Source: CAD feature listing. Evaluate the final solid. Frame: model axes, mm. A direction names the side the tool comes from. Give positions to 0.01 mm unless a question says otherwise; leave off trailing zeros. Order: outer loops, then holes, each group sorted by start corner. A loop starts at its lowest first (then second) coordinate and runs counter-clockwise, first axis right, second up. Notation, with made-up numbers: (1, 84) -> (6, 84) arc R18 ccw to (6, 117) -> close; hole circle Ø8 at (76, 42). An arc over 180 degrees is marked (long way). Use CSV: the item, a comma, the result in double quotes.
```python
from build123d import *

# Parameters (mm, degrees)
SKETCH1_W           = 80
SKETCH1_H           = 80
BOSS_EXTRUDE2_DEPTH = 10
CUT_EXTRUDE2_DEPTH  = 14
CUT_EXTRUDE3_DEPTH  = 14
CUT_EXTRUDE4_DEPTH  = 5
SCALE2_SCALE        = 0.1


with BuildPart() as part:
    # Sketch1 → Boss-Extrude2 (new body)
    with BuildSketch(Plane(origin=(0, 0, 0), x_dir=(1, 0, 0), z_dir=(0, 1, 0))):
        Rectangle(SKETCH1_W, SKETCH1_H)
    extrude(amount=BOSS_EXTRUDE2_DEPTH)

    # Sketch1<8> → Cut-Extrude2 (cut)
    with BuildSketch(Plane(origin=(0, 0, 0), x_dir=(1, 0, 0), z_dir=(0, 1, 0))):
        with BuildLine():
            Line((25, 40), (-25, 40))
            Line((-25, 40), (-25, 31.971455811))
            ThreePointArc((-25, 31.971455811), (-35.374629105, 30), (-25, 28.028544189))
            Line((-25, 28.028544189), (-25, 12.5))
            Line((-25, 12.5), (25, 12.5))
            Line((25, 12.5), (25, 28.028544189))
            ThreePointArc((25, 28.028544189), (35.374629105, 30), (25, 31.971455811))
            Line((25, 31.971455811), (25, 40))
        make_face()
    extrude(amount=CUT_EXTRUDE2_DEPTH, mode=Mode.SUBTRACT)

    # Sketch4 → Cut-Extrude3 (cut)
    with BuildSketch(Plane.XZ):
        Polygon((40, 40), (-40, 40), (-40, 25), (-38, 25), (38, 25), (40, 25), align=None)
    extrude(amount=-CUT_EXTRUDE3_DEPTH, mode=Mode.SUBTRACT)

    # Sketch4<4> → Cut-Extrude4 (cut)
    with BuildSketch(Plane.XZ):
        with BuildLine():
            Line((38, 25), (-38, 25))
            Line((-38, 25), (-38, -38))
            Line((-38, -38), (-27, -38))
            Line((-27, -38), (-25, -38))
            Line((-25, -38), (-25, -31.971455811))
            ThreePointArc((-25, -31.971455811), (-35.374629105, -30), (-25, -28.028544189))
            Line((-25, -28.028544189), (-25, -12.5))
            Line((-25, -12.5), (25, -12.5))
            Line((25, -12.5), (25, -28.028544189))
            ThreePointArc((25, -28.028544189), (35.374629105, -30), (25, -31.971455811))
            Line((25, -31.971455811), (25, -38))
            Line((25, -38), (27, -38))
            Line((27, -38), (38, -38))
            Line((38, -38), (38, 25))
        make_face()
    extrude(amount=-CUT_EXTRUDE4_DEPTH, mode=Mode.SUBTRACT)


with BuildPart() as part_1:
    # Scale2: scaled about (0, 7.105810112, -0.378714582)
    add(part.part.scale(SCALE2_SCALE).moved(Location((0, 6.395229101, -0.340843124))))


solid = part_1.part
```
1. Section query C-C on y = 6.7. Return loops of the section in (x, z), plus the area to 3 significant figures.
Answer below:
outline,"(-4, -4.34) -> (-2.5, -4.34) -> (-2.5, -4.14) -> (-3.8, -4.14) -> (-3.8, 2.16) -> (-4, 2.16) -> close; (2.5, -4.34) -> (4, -4.34) -> (4, 2.16) -> (3.8, 2.16) -> (3.8, -4.14) -> (2.5, -4.14) -> close"
area,"3.12 mm²"
2. Mould query, pull axis X, two halves, no side actions, for faces 4 (the flat face through (4, 7, -1)), 5 (the cylindrical face through (3.537, 7.142, -3.32)), 6 (the cylindrical face through (-3.537, 7.142, -3.362)), 7 (the flat face through (-4, 7, -1)). Classes: released by +X, released by -X, zero draft, split by the parting line, or undercut.
Answer below:
face 4,"released by +X"
face 5,"undercut"
face 6,"undercut"
face 7,"released by -X"
3. Pin query (flat end, axial travel): P1, Ø1.9, axis at x = -2, z = -0.5, coming from the -Y side; P2, Ø0.6, axis at x = 0, y = 7, coming from the -Z side; P3, Ø1, axis at x = 3, z = -3.34, coming from the +Y side. Return the tip coordinate at first contact, or that it passes through.
Answer below:
P1,"stops at y = 6.9"
P2,"stops at z = -1.59"
P3,"passes through"
4. Section query D-D on z = -0.5. Return loops of the section in (x, y).
Answer below:
outline,"(-4, 6.4) -> (-3.8, 6.4) -> (-3.8, 6.9) -> (3.8, 6.9) -> (3.8, 6.4) -> (4, 6.4) -> (4, 7.4) -> (-4, 7.4) -> close"
5. Ray query, line 1 along X through (y, z) = (7.05, -2.5); line 2 along X through (y, z) = (6.85, 0.5); line 3 along Z through (x, y) = (3, 7.2). Return the intervals inside material, ascending.
Answer below:
line 1,"x = -4 to -2.5, 2.5 to 4"
line 2,"x = -4 to -3.8, 3.8 to 4"
line 3,"z = -4.34 to -3.88, -2.8 to 2.16"
6. Section query B-B on x = 3. Return loops of the section in (y, z), plus the area to 3 significant figures.
Answer below:
outline,"(6.4, -4.34) -> (7.4, -4.34) -> (7.4, -3.88) -> (6.9, -3.88) -> (6.9, -4.14) -> (6.4, -4.14) -> close; (6.9, -2.8) -> (7.4, -2.8) -> (7.4, 2.16) -> (6.9, 2.16) -> close"
area,"2.81 mm²"
7. Access query for faces 1 (the flat face through (2.5, 7.1, -4)), 2 (the flat face through (0, 6.895, 0)), 3 (the flat face through (0, 7.395, 0)). Directions: +Z, -Z, +X, -X, +Y, -Y. A direction counts if a zero-diameter tool reaches every point of the face in a straight line with its end or side. Return the directions, or none.
Answer below:
face 1,"-Z, +Y, -Y"
face 2,"+Z, -Y"
face 3,"+Z, -Z, +X, -X, +Y"
8. Section query A-A on z = -2.5. Return loops of the section in (x, y).
Answer below:
outline,"(-4, 6.4) -> (-3.8, 6.4) -> (-3.8, 6.9) -> (-2.5, 6.9) -> (-2.5, 7.4) -> (-4, 7.4) -> close; (2.5, 6.9) -> (3.8, 6.9) -> (3.8, 6.4) -> (4, 6.4) -> (4, 7.4) -> (2.5, 7.4) -> close"
